Study the drawing (mm; zero at the part's minimum x, y, z) and answer. Coordinates: 2 decimals unless noted, no trailing zeros. Write each loop counter-clockwise with the first axis right and the second up, starting at its lowest first coordinate (ties: lowest second). Pieces come first, ordered by that corner, then holes. Notation, with made-up numbers: (13, 64) - (56, 64) arc R27 cw to (56, 81) - close; hole circle Ø1 at (16, 29). An arc over 180 degrees is marked (long way). One line per item, written item: value.
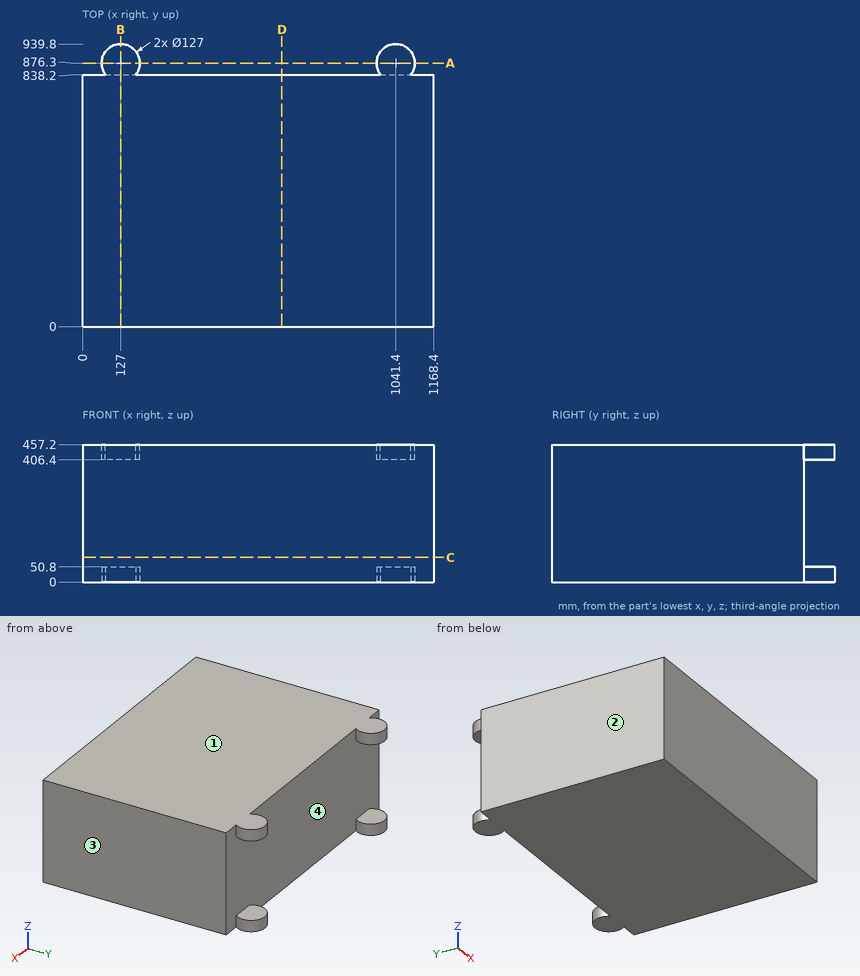
Item 1: Section C-C, the plane z = 82 is taken. Determine the outline of the cut face in (x, y), then the cut area to 3 significant figures.
Evaluation:
outline: (0, 0) - (1168.4, 0) - (1168.4, 838.2) - (0, 838.2) - close
area: 979,000 mm2
Item 2: Consider probe 1 along Y at (x, z) = (641.5, 396); probe 2 along Y at (x, z) = (1053.5, 44). Determine where each line is inside the solid, lowest interval first.
Evaluation:
probe 1: y = 0 to 838.2
probe 2: y = 0 to 938.64
Item 3: Determine the mould class of the marked faces 1, 2, 3 and 4 for opening direction X: +X half, -X half, draft (parallel to the pull), parting line (faces both ways), or undercut.
Evaluation:
face 1: draft
face 2: -X half
face 3: +X half
face 4: undercut
Item 4: Section B-B, the plane x = 127 is taken. Determine the outline of the cut face in (y, z), then the cut area to 3 significant figures.
Evaluation:
outline: (0, 0) - (939.8, 0) - (939.8, 50.8) - (838.2, 50.8) - (838.2, 406.4) - (939.8, 406.4) - (939.8, 457.2) - (0, 457.2) - close
area: 394,000 mm2
Item 5: Given pin 1 (5 mm diameter, centred on x = 749, z = 128, fed in from +Y); pin 2 (1.5 mm diameter, centred on y = 396.5, z = 74, fed in from -X), each flat-ended and moving along its own axis, determine where each tip first touches the part or whether it passes through.
Evaluation:
pin 1: stops at y = 838.2
pin 2: stops at x = 0
Item 6: Section A-A, the plane y = 876.3 is taken. Determine the outline of the cut face in (x, z), then the cut area to 3 significant figures.
Evaluation:
outline: (63.5, 0) - (190.5, 0) - (190.5, 50.8) - (63.5, 50.8) - close; (63.5, 406.4) - (190.5, 406.4) - (190.5, 457.2) - (63.5, 457.2) - close; (977.9, 0) - (1104.9, 0) - (1104.9, 50.8) - (977.9, 50.8) - close; (977.9, 406.4) - (1104.9, 406.4) - (1104.9, 457.2) - (977.9, 457.2) - close
area: 25,800 mm2
Item 7: Section D-D, the plane x = 663 is taken. Determine the outline of the cut face in (y, z), then the cut area to 3 significant figures.
Evaluation:
outline: (0, 0) - (838.2, 0) - (838.2, 457.2) - (0, 457.2) - close
area: 383,000 mm2
